Here's how the part is built. I have some questions about the finished solid (model axes, mm). A direction names the side the tool comes from. Coordinates: 2 decimals unless noted, no trailing zeros. Answer as a JSON object with one key per item and string values. Group by question number.
Q1. I'm going to push flat-ended pins straight in: pin 1 (10 mm diameter, centred on x = 695, z = 17.9, fed in from -Y); pin 2 (14.5 mm diameter, centred on x = 94.5, z = 19.5, fed in from +Y). Where does each tip first touch, or does it pass through?
Q2. I need wall thicknesses on line 1 (X direction, y = 12, z = 68); line 2 (Z direction, x = 695, y = 67); line 3 (Z direction, x = 495, y = 76). Which ranges of each line are inside material? Lowest first, please.
Q3. Thinking about a two-plate mould opening in X: for faces 3 (the flat face through (350, 83, 44)), 4 (the cylindrical face through (703.314, 77.577, 21.347)), 5 (the flat face through (710, 41, 44)), which applies, released by +X, released by -X, zero draft, split by the parting line, or undercut?
Q4. On a 3-axis mill with a long thin cutter (end or side, diameter ignored), from which of +Z, -Z, +X, -X, +Y, -Y can I reach the whole of each face in a straight line? I mean faces 1 (the cylindrical face through (503.584, 77.577, 65.197)), 2 (the flat face through (0, 41, 44)). Say none if no direction works.
```python
from build123d import *

# Parameters (mm, degrees)
SKETCH1_W                                            = 710
SKETCH1_H                                            = 83
BOSS_EXTRUDE1_DEPTH                                  = 88.9
M8_TAPPED_HOLE1_D                                    = 6.8
M8_TAPPED_HOLE1_DEPTH                                = 32.99
M8_TAPPED_HOLE1_TIP                                  = 2.042926105
CBORE_FOR_M10_HEX_SOCKET_HEAD_CAP_SCREW1_D           = 11
CBORE_FOR_M10_HEX_SOCKET_HEAD_CAP_SCREW1_CBORE_D     = 18
CBORE_FOR_M10_HEX_SOCKET_HEAD_CAP_SCREW1_CBORE_DEPTH = 11
M6_TAPPED_HOLE1_D                                    = 5
M6_TAPPED_HOLE1_DEPTH                                = 21.35
M6_TAPPED_HOLE1_TIP                                  = 1.502151548
M8_TAPPED_HOLE2_D                                    = 6.8
M8_TAPPED_HOLE2_DEPTH                                = 32.99
M8_TAPPED_HOLE2_TIP                                  = 2.042926105


with BuildPart() as part:
    # Sketch1 → Boss-Extrude1 (new body)
    with BuildSketch(Plane.XY):
        with Locations((355, 41.5)):
            Rectangle(SKETCH1_W, SKETCH1_H)
    extrude(amount=BOSS_EXTRUDE1_DEPTH)

    # M8 Tapped Hole1
    with Locations(Plane(origin=(0, 83, 0), x_dir=(1, 0, 0), z_dir=(0, 1, 0))):
        with Locations((95, -67.9), (195, -67.9), (295, -17.9), (395, -67.9), (495, -17.9), (595, -67.9), (695, -67.9)):
            Hole(M8_TAPPED_HOLE1_D / 2, depth=M8_TAPPED_HOLE1_DEPTH)
            with Locations((0, 0, -(M8_TAPPED_HOLE1_DEPTH + M8_TAPPED_HOLE1_TIP / 2))):  # 118° drill point
                Cone(0, M8_TAPPED_HOLE1_D / 2, M8_TAPPED_HOLE1_TIP, mode=Mode.SUBTRACT)

    # CBORE for M10 Hex Socket Head Cap Screw1 (through all)
    with Locations(Plane(origin=(0, 83, 0), x_dir=(1, 0, 0), z_dir=(0, 1, 0))):
        with Locations((695, -17.9), (495, -67.9), (295, -67.9), (95, -17.9)):
            CounterBoreHole(CBORE_FOR_M10_HEX_SOCKET_HEAD_CAP_SCREW1_D / 2, CBORE_FOR_M10_HEX_SOCKET_HEAD_CAP_SCREW1_CBORE_D / 2, CBORE_FOR_M10_HEX_SOCKET_HEAD_CAP_SCREW1_CBORE_DEPTH)

    # M6 Tapped Hole1
    with Locations(Plane(origin=(0, 83, 0), x_dir=(1, 0, 0), z_dir=(0, 1, 0))):
        with Locations((16, -55.9), (43, -55.9)):
            Hole(M6_TAPPED_HOLE1_D / 2, depth=M6_TAPPED_HOLE1_DEPTH)
            with Locations((0, 0, -(M6_TAPPED_HOLE1_DEPTH + M6_TAPPED_HOLE1_TIP / 2))):  # 118° drill point
                Cone(0, M6_TAPPED_HOLE1_D / 2, M6_TAPPED_HOLE1_TIP, mode=Mode.SUBTRACT)

    # M8 Tapped Hole2
    with Locations(Plane.XY.offset(88.9)):
        with Locations((246.5, 43), (446.5, 43), (632.5, 43)):
            Hole(M8_TAPPED_HOLE2_D / 2, depth=M8_TAPPED_HOLE2_DEPTH)
            with Locations((0, 0, -(M8_TAPPED_HOLE2_DEPTH + M8_TAPPED_HOLE2_TIP / 2))):  # 118° drill point
                Cone(0, M8_TAPPED_HOLE2_D / 2, M8_TAPPED_HOLE2_TIP, mode=Mode.SUBTRACT)


solid = part.part
```
Result set:
{
 "1": {"pin 1": "passes through", "pin 2": "stops at y = 72"},
 "2": {"line 1": "x = 0 to 289.5, 300.5 to 489.5, 500.5 to 710", "line 2": "z = 0 to 12.4, 23.4 to 64.5, 71.3 to 88.9", "line 3": "z = 0 to 14.5, 21.3 to 58.9, 76.9 to 88.9"},
 "3": {"face 3": "zero draft", "face 4": "undercut", "face 5": "released by +X"},
 "4": {"face 1": "+Y", "face 2": "+Z, -Z, -X, +Y, -Y"}
}
